Input: dimensioned drawing with shaded views. Units: mm. Origin: part minimum x, y, z. A direction names the side the tool comes from. Coordinates: 2 decimals unless noted, no trailing zeros. Order: outer loops, then holes, each group sorted by start corner. A loop starts at its lowest first (then second) coordinate and runs counter-clockwise, first axis right, second up. Notation, with made-up numbers: (-40, 70.25) -> (-5, 70.25) arc R22 cw to (-5, 109.25) -> close; hole circle Ø9 at (63.5, 42.5). An arc over 180 degrees is marked (long way). Answer as CSV lines item,"result".
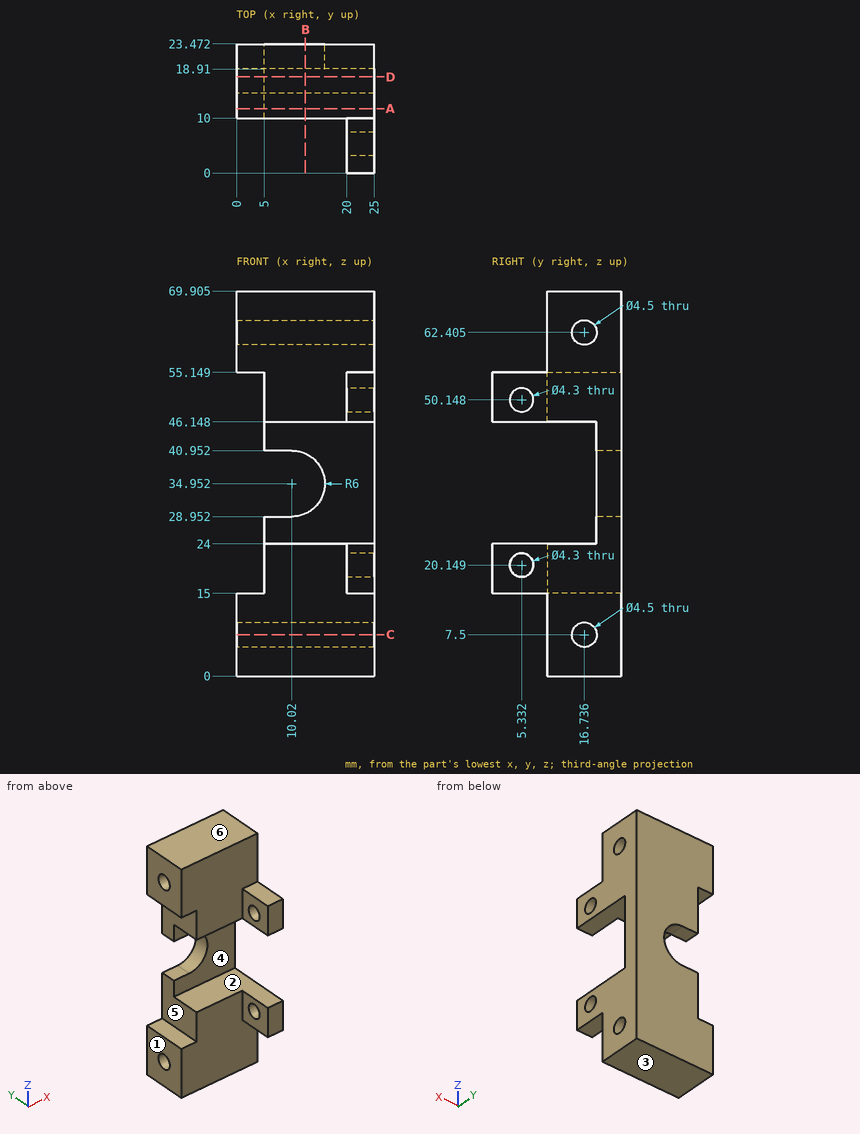
1. Cut plane A-A (y = 11.75). Return the cut outline in (x, z) (1 decimal).
Findings:
outline,"(0, 0) -> (25, 0) -> (25, 24) -> (5, 24) -> (5, 15) -> (0, 15) -> close; (0, 55.1) -> (5, 55.1) -> (5, 46.1) -> (25, 46.1) -> (25, 69.9) -> (0, 69.9) -> close"
2. Cut plane D-D (y = 17.5). Return the cut outline in (x, z) (1 decimal).
Findings:
outline,"(0, 0) -> (25, 0) -> (25, 5.4) -> (0, 5.4) -> close; (0, 9.6) -> (25, 9.6) -> (25, 24) -> (5, 24) -> (5, 15) -> (0, 15) -> close; (0, 55.1) -> (5, 55.1) -> (5, 46.1) -> (25, 46.1) -> (25, 60.3) -> (0, 60.3) -> close; (0, 64.5) -> (25, 64.5) -> (25, 69.9) -> (0, 69.9) -> close"
3. Mould query, pull axis Z, two halves, no side actions, for the marked faces 1, 2 and 3. Classes: released by +Z, released by -Z, zero draft, split by the parting line, or undercut.
Findings:
face 1,"zero draft"
face 2,"undercut"
face 3,"released by -Z"
4. Ray query, line 1 along Y through (x, z) = (19.5, 7.5) (1 decimal); line 2 along Z through (x, y) = (10, 17) (1 decimal); line 3 along Z through (x, y) = (18.5, 11) (1 decimal). Return the intervals inside material, ascending.
Findings:
line 1,"y = 10 to 14.5, 19 to 23.5"
line 2,"z = 0 to 5.3, 9.7 to 24, 46.1 to 60.2, 64.6 to 69.9"
line 3,"z = 0 to 24, 46.1 to 69.9"
5. Contact query for flat-ended pins moving along their axis: pin 1 (2.5 mm diameter, centred on y = 5.33, z = 50.15, fed in from +X); pin 2 (10 mm diameter, centred on y = 5, z = 42.5, fed in from -X); pin 3 (2.5 mm diameter, centred on x = 23.5, y = 4, fed in from -Z); pin 4 (5.5 mm diameter, centred on x = 22.5, y = 4.5, fed in from +Z). Output: stop coordinate, or through.
Findings:
pin 1,"passes through"
pin 2,"stops at x = 20"
pin 3,"stops at z = 15"
pin 4,"stops at z = 55.15"
6. Reachability of the marked faces 4, 5 and 6 from +Z, -Z, +X, -X, +Y, -Y: full face, straight path, thin tool, end or side. Return the list, or none.
Findings:
face 4,"+X, -X, -Y"
face 5,"-X, +Y, -Y"
face 6,"+Z, +X, -X, +Y, -Y"
7. Cut plane C-C (z = 7.5). Return the cut outline in (x, y) (1 decimal).
Findings:
outline,"(0, 10) -> (25, 10) -> (25, 14.5) -> (0, 14.5) -> close; (0, 19) -> (25, 19) -> (25, 23.5) -> (0, 23.5) -> close"
8. Cut plane B-B (x = 12.5). State how many separate pieces and enclosed holes the cut face has, plus the area to 3 significant figures.
Findings:
separate pieces,"2"
enclosed holes,"2"
area,"663 mm2"
